Autodesk Fusion 360 part; units mm, degrees
sketch "Esquisse1" plane through (0, 0, 0) normal (0, 1, 0) x (1, 0, 0)
  line L0 (0, 0) -> (-160, 0)
  line L1 (-160, 0) -> (-160, 3)
  line L2 (-160, 3) -> (0, 3)
  line L3 (0, 3) -> (0, 0)
  line L4 (0, 7) -> (-160, 7)
  line L5 (-160, 7) -> (-160, 10)
  line L6 (-160, 10) -> (0, 10)
  line L7 (0, 10) -> (0, 7)
  line L8 (-137.5, 3) -> (-162.5, 3)
  line L9 (-162.5, 3) -> (-162.5, 7)
  line L10 (-162.5, 7) -> (-137.5, 7)
  line L11 (-137.5, 7) -> (-137.5, 3)
  line L12 (-22.5, 7) -> (2.5, 7)
  line L13 (2.5, 7) -> (2.5, 3)
  line L14 (2.5, 3) -> (-22.5, 3)
  line L15 (-22.5, 3) -> (-22.5, 7)
  dimension "d1" = 160
  dimension "d2" = 3
  dimension "d3" = 160
  dimension "d4" = 3
  dimension "d5" = 4
  dimension "d6" = 25
  dimension "d7" = 2.5
  dimension "d8" = 4
  dimension "d9" = 4
  dimension "d10" = 25
  dimension "d11" = 2.5
extrude "Extrusion1" add sketch "Esquisse1" along normal blind 50 contours L0 L1 L2 L3 L8 L14 | L2 L4 L12 L13 L14 L15 | L2 L4 L8 L9 L10 L11 | L4 L5 L6 L7 L10 L12
sketch "Esquisse2" plane through (0, 0, 0) normal (0, -1, 0) x (1, 0, 0)
  line L0 (-22.5, -3) -> (-22.5, -7)
  line L1 (-22.5, -7) -> (-137.5, -7)
  line L2 (-137.5, -7) -> (-137.5, -3)
  line L3 (-137.5, -3) -> (-22.5, -3)
  line L4 (2.5, -7) -> (2.5, -3)
  line L5 (2.5, -3) -> (0, -3)
  line L6 (0, -3) -> (0, 0)
  line L7 (0, 0) -> (-160, 0)
  line L8 (-160, 0) -> (-160, -3)
  line L9 (-160, -3) -> (-162.5, -3)
  line L10 (-162.5, -3) -> (-162.5, -7)
  line L11 (-162.5, -7) -> (-160, -7)
  line L12 (-160, -7) -> (-160, -10)
  line L13 (-160, -10) -> (0, -10)
  line L14 (0, -10) -> (0, -7)
  line L15 (0, -7) -> (2.5, -7)
  line L16 (-22.5, -3) -> (2.5, -3)
  line L17 (2.5, -3) -> (2.5, -7)
  line L18 (2.5, -7) -> (-22.5, -7)
  line L19 (-22.5, -7) -> (-22.5, -3)
  line L20 (-137.5, -7) -> (-162.5, -7)
  line L21 (-162.5, -7) -> (-162.5, -3)
  line L22 (-162.5, -3) -> (-137.5, -3)
  line L23 (-137.5, -3) -> (-137.5, -7)
extrude "Extrusion2" cut sketch "Esquisse2" against normal blind 4 contours L0 L4 L5 L15 L16 L17 L18 L19 | L2 L9 L10 L11 L20 L21 L22 L23
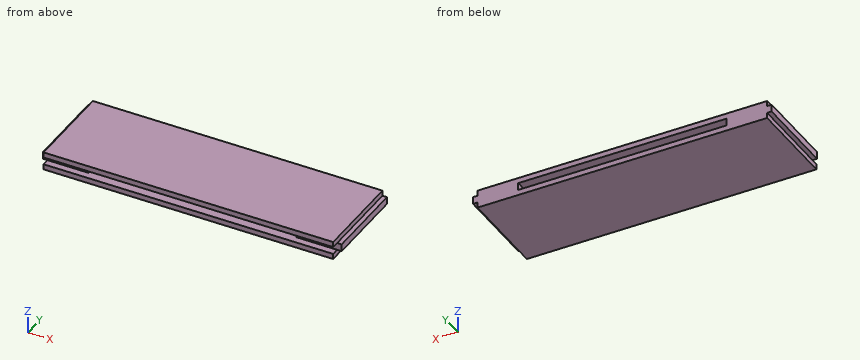
Source: CAD feature listing. Evaluate the final solid. Frame: model axes, mm. Round coordinates to 2 decimals unless told otherwise and drop trailing zeros. Loops run counter-clockwise (first coordinate to the right, second up) from the corner with the lowest first, then second, coordinate; pieces in that order, holes last. Notation, with made-up numbers: M 24.25,80 L 30.25,80 A24 ccw 30.25,105 Z; hole C -4.75,69 d1. An arc over 180 degrees is marked long. Put each result on its own line as item: value.
(1) First-contact query: pin 1 (0.8 mm diameter, centred on x = 2, y = 19, fed in from -Z); pin 2 (1.2 mm diameter, centred on x = 1.5, y = 26, fed in from +Z); pin 3 (1.5 mm diameter, centred on y = 20, z = -1.5, fed in from +X); pin 4 (1 mm diameter, centred on x = -84, z = -6, fed in from +Y). Flat tips, straight axial feed; report the tip coordinate or a pass-through.
Solutions:
pin 1: z = -7
pin 2: z = -3
pin 3: x = 0
pin 4: through
(2) Ray query, line 1 (Z direction, x = -106, y = 7); line 2 (X direction, y = 4.5, z = -6.75); line 3 (X direction, y = 14, z = -7.5). Return the intervals inside material, ascending. Write a range as [from, to].
Solutions:
line 1: [-10, -7], [-3, 0]
line 2: [-162.5, -137.5], [-22.5, 2.5]
line 3: [-160, 0]
(3) Section A-A, the plane x = -26. Return loops of the section in (y, z).
Solutions:
outline: M 0,-10 L 50,-10 L 50,-7 L 0,-7 Z; M 0,-3 L 50,-3 L 50,0 L 0,0 Z
(4) Section C-C, the plane y = 26.5. Return loops of the section in (x, z).
Solutions:
outline: M -162.5,-7 L -160,-7 L -160,-10 L 0,-10 L 0,-7 L 2.5,-7 L 2.5,-3 L 0,-3 L 0,0 L -160,0 L -160,-3 L -162.5,-3 Z; hole M -137.5,-7 L -22.5,-7 L -22.5,-3 L -137.5,-3 Z
(5) Section B-B, the plane z = -5. Return loops of the section in (x, y).
Solutions:
outline: M -162.5,4 L -137.5,4 L -137.5,50 L -162.5,50 Z; M -22.5,4 L 2.5,4 L 2.5,50 L -22.5,50 Z
